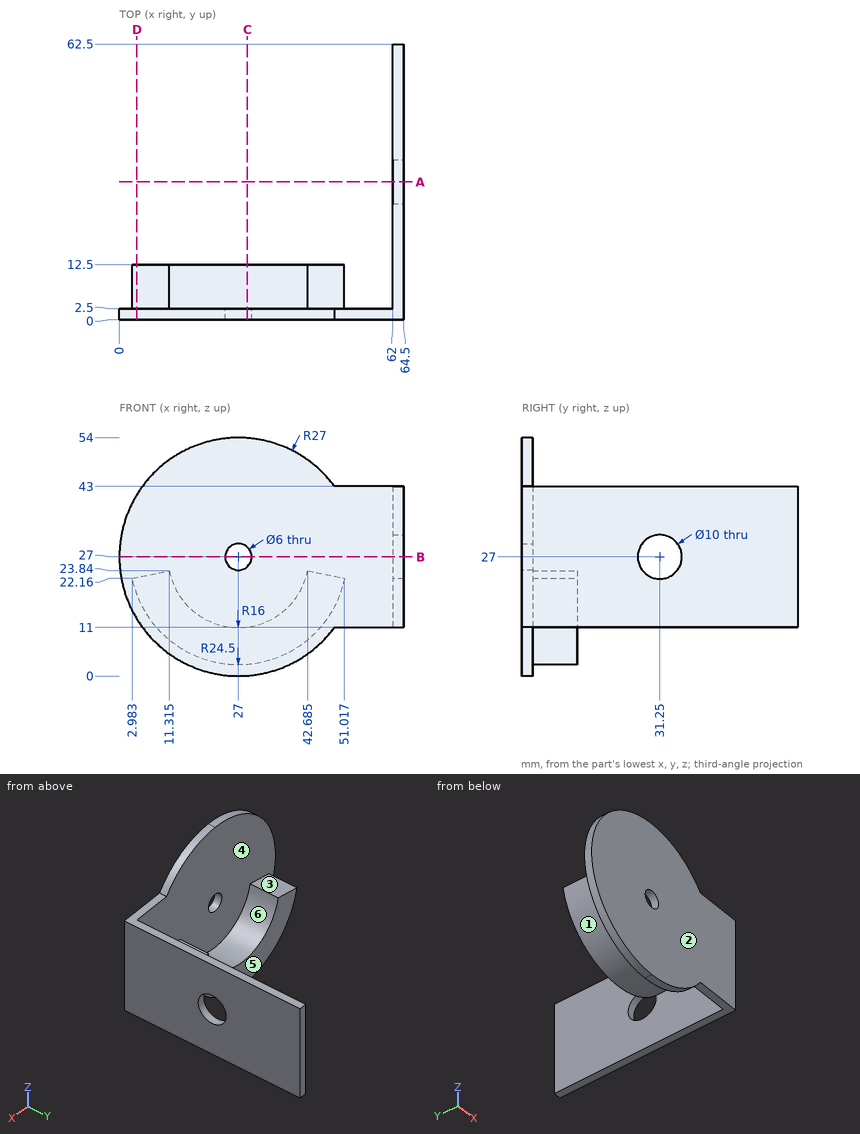
The drawing under review shows one solid part. Ordinate dimensions are in mm from its lowest x, y, z. A direction names the side the tool comes from. Give positions to 0.01 mm unless a question says otherwise; leave off trailing zeros. Loops run counter-clockwise (first coordinate to the right, second up) from the corner with the lowest first, then second, coordinate; pieces in that order, holes last. Notation, with made-up numbers: M 77.25,65 L 107.25,65 A21 cw 107.25,104 Z; hole C 22.5,-2 d5. An arc over 180 degrees is marked long. Return JSON: item names as keys, results as strings. Group by question number.
Item 1: Mouldability with a two-part tool opening along X and no side actions: class the marked faces 3, 4, 5 and 6 as released by +X, released by -X, zero draft, split by the parting line, or undercut.
Item 2: Tool access review of the marked faces 1 and 2: name each direction out of +Z, -Z, +X, -X, +Y, -Y from which nothing blocks a thin tool from reaching the whole face with its end or side.
Item 3: Insertion check: pin 1 Ø1.5 at (x, y) = (43, 9.5) entering from +Z; pin 2 Ø16 at (y, z) = (31.25, 27) entering from +X; pin 3 Ø8 at (y, z) = (12.5, 23) entering from -X; pin 4 Ø17 at (x, z) = (25, 8.5) entering from +Y. Each pin has a flat end and moves straight along its axis. Give the tip position at first contact, or say it passes through.
Item 4: We need section D-D (x = 4). Give the boundary of the cut face in (y, z) (1 decimal), and give its area (3 significant figures).
Item 5: We need section C-C (x = 29). Give the boundary of the cut face in (y, z) (1 decimal), and give its area (3 significant figures).
Item 6: We need section B-B (z = 27). Give the boundary of the cut face in (x, y), and give its area (3 significant figures).
Item 7: We need section A-A (y = 31.25). Give the boundary of the cut face in (x, z).
Item 8: For probe 1 along Z at (x, y) = (63, 31); probe 2 along Y at (x, z) = (63, 27); probe 3 along X at (y, z) = (0.85, 27), list the stretches that pass through material, from the lowest coordinate up.
Output:
{
 "1": {"face 3": "released by -X", "face 4": "undercut", "face 5": "zero draft", "face 6": "undercut"},
 "2": {"face 1": "-Z, +Y", "face 2": "+Z, -Z, +X, -X, -Y"},
 "3": {"pin 1": "stops at z = 23.84", "pin 2": "stops at x = 64.5", "pin 3": "stops at x = 2.98", "pin 4": "stops at y = 12.5"},
 "4": {"outline": "M 0,12.9 L 2.5,12.9 L 2.5,18.6 L 12.5,18.6 L 12.5,22.4 L 2.5,22.4 L 2.5,41.1 L 0,41.1 Z", "area": "109 mm^2"},
 "5": {"outline": "M 0,0.1 L 2.5,0.1 L 2.5,2.6 L 12.5,2.6 L 12.5,11.1 L 2.5,11.1 L 2.5,24.8 L 0,24.8 Z; M 0,29.2 L 2.5,29.2 L 2.5,53.9 L 0,53.9 Z", "area": "209 mm^2"},
 "6": {"outline": "M 0,0 L 24,0 L 24,2.5 L 0,2.5 Z; M 30,0 L 64.5,0 L 64.5,26.25 L 62,26.25 L 62,2.5 L 30,2.5 Z; M 62,36.25 L 64.5,36.25 L 64.5,62.5 L 62,62.5 Z", "area": "271 mm^2"},
 "7": {"outline": "M 62,11 L 64.5,11 L 64.5,22 L 62,22 Z; M 62,32 L 64.5,32 L 64.5,43 L 62,43 Z"},
 "8": {"probe 1": "z = 11 to 22.01, 31.99 to 43", "probe 2": "y = 0 to 26.25, 36.25 to 62.5", "probe 3": "x = 0 to 24, 30 to 64.5"}
}
